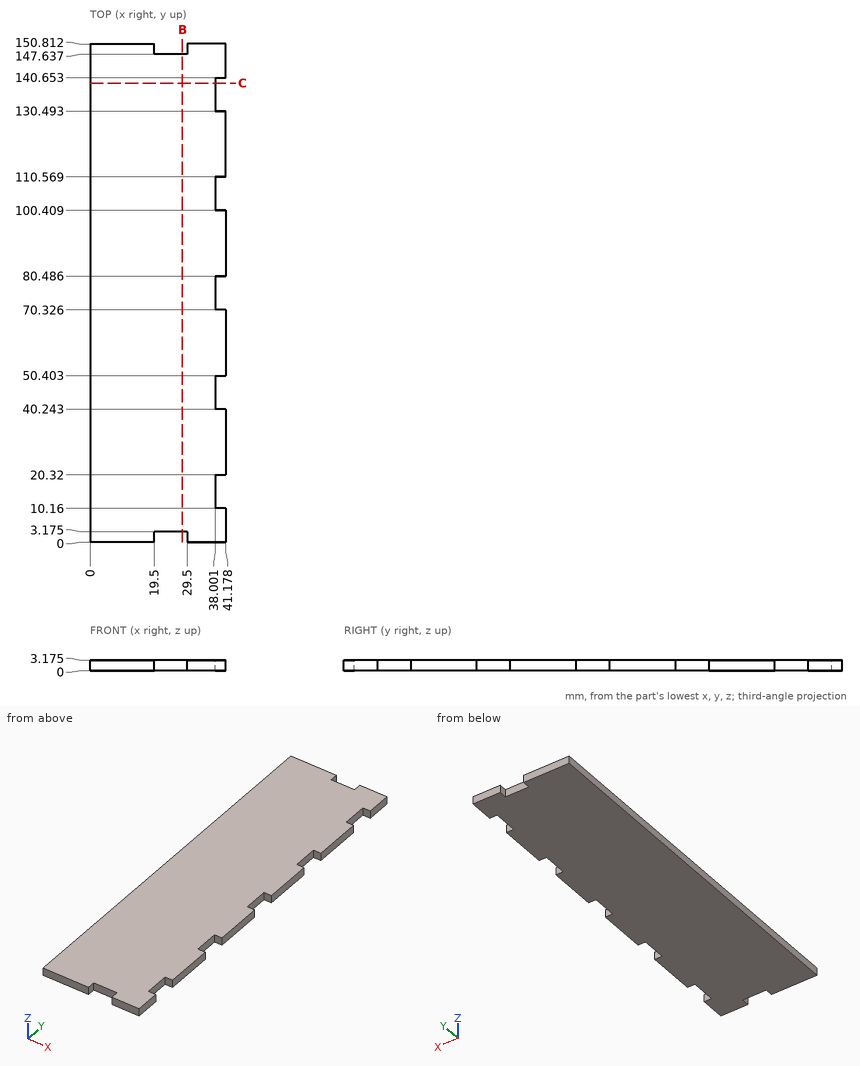
Part print with two shaded views. Sizes in mm from the minimum x, y, z corner. Give positions to 0.01 mm unless a question says otherwise; leave off trailing zeros. Order: outer loops, then holes, each group sorted by start corner. A loop starts at its lowest first (then second) coordinate and runs counter-clockwise, first axis right, second up.
1) Saw through at C-C, the plane y = 139. Write the cut outline in (x, z) (1 decimal), then the cut area to 3 significant figures.
2) Wall check: probe 1 along X at (y, z) = (14, 0.65); probe 2 along Y at (x, z) = (24, 1.3) (1 decimal). Give the ranges that are in metal, low to high.
3) Pin check, flat tip, straight feed: pin 1 (1.6 mm diameter, centred on y = 77.5, z = 1.5, fed in from +X). Stop position of the tip, or through.
4) Saw through at B-B, the plane x = 28. Write the cut outline in (y, z) (1 decimal).
Computed:
1. outline: (0, 0) - (38, 0) - (38, 3.2) - (0, 3.2) - close
1. area: 121 mm2
2. probe 1: x = 0 to 38
2. probe 2: y = 3.2 to 147.6
3. pin 1: stops at x = 38
4. outline: (3.2, 0) - (147.6, 0) - (147.6, 3.2) - (3.2, 3.2) - close
